```python
from build123d import *

# Parameters (mm, degrees)
F1_DEPTH = 20
F0_R     = 1.6
F2_DEPTH = 15
F4_R     = 3
F5_DEPTH = 85


with BuildPart() as f1:
    # F0 (on Top) → F1 (new body)
    with BuildSketch(Plane.XY):
        with BuildLine():
            Line((9, 82), (9, 78))
            ThreePointArc((9, 78), (14.6568542495, 80.3431457505), (17, 86))
            ThreePointArc((17, 86), (5.9385325411, 93.3910362601), (3.3431457505, 80.3431457505))
            Line((3.3431457505, 80.3431457505), (6.1715728753, 83.1715728753))
            ThreePointArc((6.1715728753, 83.1715728753), (5, 86), (6.1715728753, 88.8284271247))
            ThreePointArc((6.1715728753, 88.8284271247), (10.5307337295, 89.69551813), (13, 86))
            ThreePointArc((13, 86), (12.69551813, 84.4692662705), (11.8284271247, 83.1715728753))
            ThreePointArc((11.8284271247, 83.1715728753), (10.5307337295, 82.30448187), (9, 82))
        make_face()
        with BuildLine():
            ThreePointArc((3.3431457505, 80.3431457505), (5.9385325411, 78.6089637399), (9, 78))
            Line((9, 78), (9, 82))
            ThreePointArc((9, 82), (7.4692662705, 82.30448187), (6.1715728753, 83.1715728753))
            Line((6.1715728753, 83.1715728753), (3.3431457505, 80.3431457505))
        make_face()
    extrude(amount=F1_DEPTH)

    # F0 (on Top) → F2 (join)
    with BuildSketch(Plane.XY):
        with BuildLine():
            ThreePointArc((9, 76.3), (17.2071692051, 91.4977753902), (0, 90))
            Line((0, 90), (0, 0))
            Line((0, 0), (18, 0))
            Line((18, 0), (18, 8))
            Line((18, 8), (9, 16))
            Line((9, 16), (9, 46))
            Line((9, 46), (9, 76.3))
        make_face()
        with Locations((3, 4)):
            Circle(F0_R, mode=Mode.SUBTRACT)
        with BuildLine():
            ThreePointArc((16.6, 4), (15, 2.4), (13.4, 4))
            ThreePointArc((13.4, 4), (15, 5.6), (16.6, 4))
        make_face(mode=Mode.SUBTRACT)
        with BuildLine():
            ThreePointArc((17, 86), (14.6568542495, 80.3431457505), (9, 78))
            ThreePointArc((9, 78), (5.9385325411, 78.6089637399), (3.3431457505, 80.3431457505))
            ThreePointArc((3.3431457505, 80.3431457505), (5.9385325411, 93.3910362601), (17, 86))
        make_face(mode=Mode.SUBTRACT)
    extrude(amount=F2_DEPTH)

    # F4 (on face) → F5 (cut)
    with BuildSketch(Plane.XZ):
        with Locations((5.5, 7.5)):
            Circle(F4_R)
    extrude(amount=-F5_DEPTH, mode=Mode.SUBTRACT)


solid = f1.part
```
Could you check a few things on this model? Use its own coordinates, in mm. A direction names the side the tool comes from. Round coordinates to 2 decimals unless told otherwise and drop trailing zeros. Loops run counter-clockwise (first coordinate to the right, second up) from the corner with the lowest first, then second, coordinate; pieces in that order, holes last. Notation, with made-up numbers: M 33,26.25 L 46,26.25 A7 ccw 46,37.25 Z; hole C -20,-24.75 d2. An arc over 180 degrees is marked long. Put each result on its own line as item: value.
Q1. For pin 1 (3.5 mm diameter, centred on x = 15, y = 4, fed in from +Z); pin 2 (6.5 mm diameter, centred on y = 3.5, z = 8, fed in from +X); pin 3 (2 mm diameter, centred on y = 19.5, z = 11.5, fed in from +X), each with a flat end and sliding along its axis, tell me the tip position at first contact or that it passes through.
Check result:
pin 1: z = 15
pin 2: x = 18
pin 3: x = 9
Q2. I need wall thicknesses on probe 1 along Z at (x, y) = (5.5, 17); probe 2 along Y at (x, z) = (15, 11); probe 3 along Y at (x, z) = (11.25, 11). Which ranges of each line are inside material? Lowest first, please.
Check result:
probe 1: 0 to 4.5, 10.5 to 15
probe 2: 0 to 2.4, 5.6 to 10.67, 78.34 to 93.88
probe 3: 0 to 14, 76.56 to 82.69, 89.31 to 95.66
Q3. Imagine slicing it at D-D (z = 7.5). Write out the boundary of the cut face in (x, y), then the cut area to 3 significant figures.
Check result:
outline: M 0,0 L 2.5,0 L 2.5,2.48 A1.6 cw 2.5,5.52 L 2.5,85 L 5.13,85 A4 cw long 8.5,82.03 L 8.5,0 L 18,0 L 18,8 L 9,16 L 9,76.3 A9.81 ccw long 0,90 Z; hole C 15,4 d3.2
area: 544 mm2
Q4. Imagine slicing it at B-B (x = 7). Write out the boundary of the cut face in (y, z), then the cut area to 3 significant figures.
Check result:
outline: M 0,0 L 82.54,0 L 82.54,4.9 L 0,4.9 Z; M 0,10.1 L 82.54,10.1 L 82.54,20 L 78.25,20 L 78.25,15 L 0,15 Z; M 89.46,0 L 95.71,0 L 95.71,15 L 93.75,15 L 93.75,20 L 89.46,20 Z
area: 946 mm2
Q5. Imagine slicing it at C-C (y = 84). Write out the boundary of the cut face in (x, z).
Check result:
outline: M 0,0 L 5.54,0 L 5.54,4.5 A3 cw long 5.54,10.5 L 5.54,20 L 1.25,20 L 1.25,15 L 0,15 Z; M 12.46,0 L 18.59,0 L 18.59,15 L 16.75,15 L 16.75,20 L 12.46,20 Z
Q6. Thinking about a two-plate mould opening in X: for faces 1 (the face through (0, 46, 7)), 2 (the face through (4, 85, 8)), 3 (the face through (9, 46, 7)), 4 (the face through (8.36, 41.9, 8.4)), which applies, released by +X, released by -X, zero draft, split by the parting line, or undercut?
Check result:
face 1: released by -X
face 2: undercut
face 3: released by +X
face 4: undercut
Q7. On a 3-axis mill with a long thin cutter (end or side, diameter ignored), from which of +Z, -Z, +X, -X, +Y, -Y can I reach the whole of each face in a straight line? I mean faces 5 (the face through (13.563, 11.944, 7.395)), 6 (the face through (18, 4, 7)), 7 (the face through (17.366, 91.248, 7.395)). Say none if no direction works.
Check result:
face 5: +Z, -Z, +X
face 6: +Z, -Z, +X, -Y
face 7: +Z, -Z
Q8. Imagine slicing it at A-A (y = 17). Write out the boundary of the cut face in (x, z), then the cut area to 3 significant figures.
Check result:
outline: M 0,0 L 9,0 L 9,15 L 0,15 Z; hole C 5.5,7.5 d6
area: 107 mm2
